Check sheet for the drawn part. Datum: minimum x, y, z corner. Units: mm. Give positions to 0.01 mm unless a question says otherwise; leave off trailing zeros. Order: outer loops, then holes, each group sorted by start corner. A loop starts at its lowest first (then second) coordinate and runs counter-clockwise, first axis right, second up.
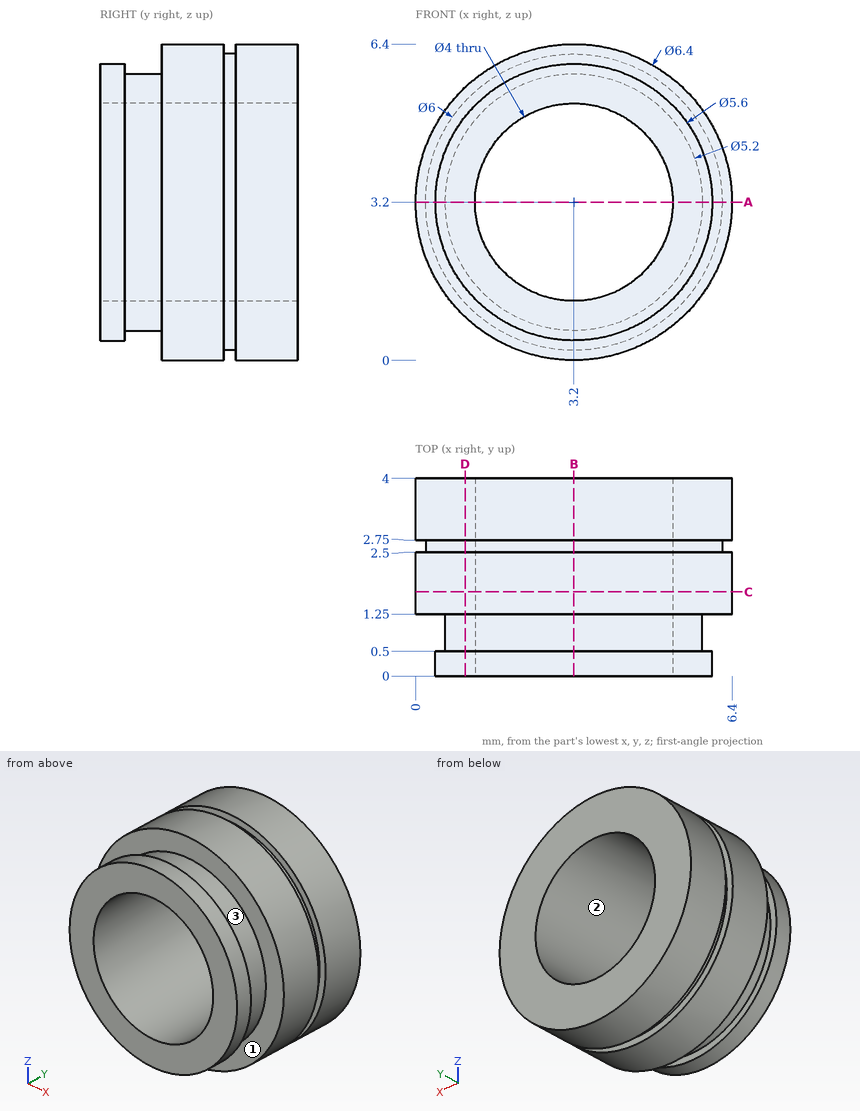
Item 1: Draft check along Z on the marked faces 1, 2 and 3. Enter one of: released by +Z, released by -Z, zero draft, split by the parting line, or undercut.
Reported:
face 1: zero draft
face 2: undercut
face 3: split by the parting line
Item 2: Sectioned sample at D-D (x = 1). Enter the section's corners in (y, z), and give its area (3 significant figures).
Reported:
outline: (0, 1.47) - (0.5, 1.47) - (0.5, 1.81) - (1.25, 1.81) - (1.25, 0.88) - (2.5, 0.88) - (2.5, 1.16) - (2.75, 1.16) - (2.75, 0.88) - (4, 0.88) - (4, 5.52) - (2.75, 5.52) - (2.75, 5.24) - (2.5, 5.24) - (2.5, 5.52) - (1.25, 5.52) - (1.25, 4.59) - (0.5, 4.59) - (0.5, 4.93) - (0, 4.93) - close
area: 16.4 mm2
Item 3: Scan lines: L1, parallel to X at y = 1.2, z = 3.2; L2, parallel to Y at x = 3.25, z = 0.5; L3, parallel to Z at x = 3.2, y = 2.1. Record each from-to range of solid material in increasing order.
Reported:
L1: x = 0.6 to 1.2, 5.2 to 5.8
L2: y = 0 to 0.5, 1.25 to 4
L3: z = 0 to 1.2, 5.2 to 6.4
Item 4: Sectioned sample at B-B (x = 3.2). Enter the section's corners in (y, z), and give its area (3 significant figures).
Reported:
outline: (0, 0.4) - (0.5, 0.4) - (0.5, 0.6) - (1.25, 0.6) - (1.25, 0) - (2.5, 0) - (2.5, 0.2) - (2.75, 0.2) - (2.75, 0) - (4, 0) - (4, 1.2) - (0, 1.2) - close; (0, 5.2) - (4, 5.2) - (4, 6.4) - (2.75, 6.4) - (2.75, 6.2) - (2.5, 6.2) - (2.5, 6.4) - (1.25, 6.4) - (1.25, 5.8) - (0.5, 5.8) - (0.5, 6) - (0, 6) - close
area: 8.20 mm2
Item 5: Sectioned sample at A-A (z = 3.2). Enter the section's corners in (x, y), and give its area (3 significant figures).
Reported:
outline: (0, 1.25) - (0.6, 1.25) - (0.6, 0.5) - (0.4, 0.5) - (0.4, 0) - (1.2, 0) - (1.2, 4) - (0, 4) - (0, 2.75) - (0.2, 2.75) - (0.2, 2.5) - (0, 2.5) - close; (5.2, 0) - (6, 0) - (6, 0.5) - (5.8, 0.5) - (5.8, 1.25) - (6.4, 1.25) - (6.4, 2.5) - (6.2, 2.5) - (6.2, 2.75) - (6.4, 2.75) - (6.4, 4) - (5.2, 4) - close
area: 8.20 mm2
Item 6: Gauge pin test, flat end, axial feed: pin 1 (1 mm diameter, centred on x = 4, y = 2.5, fed in from +Z). Record the tip position at first contact, or that the pin passes through.
Reported:
pin 1: stops at z = 6.39
Item 7: Sectioned sample at C-C (y = 1.7). Enter the section's corners in (x, z).
Reported:
outline: circle Ø6.4 at (3.2, 3.2); hole circle Ø4 at (3.2, 3.2)
